```python
from build123d import *

# Parameters (mm, degrees)
F0_R     = 1.6
F0_R_2   = 1.7
F0_R_3   = 11.25
F1_DEPTH = 10
F2_R     = 2


# Not quite as in the source:
# - a feature of the source that left no trace in its solid (it failed there, or was rolled back) is left out


with BuildPart() as f1:
    # F0 (on Front) → F1 (new body)
    with BuildSketch(Plane.XZ):
        with BuildLine():
            Line((11.2397133785, 19.9999894063), (-11.2602985395, 19.9999894063))
            ThreePointArc((-11.2602985395, 19.9999894063), (-18.3350043941, 17.0674173026), (-21.2602932426, 9.9896968203))
            Line((-21.2602932426, 9.9896968203), (-21.229426084, -19.9999894063))
            Line((-21.229426084, -19.9999894063), (-43.3949531186, -19.9999894063))
            Line((-43.3949531186, -19.9999894063), (-43.3949531186, -29.9999894063))
            Line((-43.3949531186, -29.9999894063), (43.3949531186, -29.9999894063))
            Line((43.3949531186, -29.9999894063), (43.3949531186, -19.9999894063))
            Line((43.3949531186, -19.9999894063), (21.2705964277, -19.9999894063))
            Line((21.2705964277, -19.9999894063), (21.2397080816, 10.0102819922))
            ThreePointArc((21.2397080816, 10.0102819922), (18.3071412749, 17.0746952609), (11.2397133785, 19.9999894063))
        make_face()
        with Locations((-15.6323080096, -17.1999894063)):
            Circle(F0_R, mode=Mode.SUBTRACT)
        with Locations((15.6677115429, -17.1999961863)):
            Circle(F0_R, mode=Mode.SUBTRACT)
        with Locations((-15.6645237988, 14.0999894063)):
            Circle(F0_R_2, mode=Mode.SUBTRACT)
        Circle(F0_R_3, mode=Mode.SUBTRACT)
        with Locations((15.629426084, 14.0999894063)):
            Circle(F0_R, mode=Mode.SUBTRACT)
    extrude(amount=F1_DEPTH)

    # F2
    f2_edges = [f1.edges().sort_by_distance(p)[0] for p in [
        (21.270596, -5, -19.999989),
        (-21.229426, -5, -19.999989),
    ]]
    fillet(f2_edges, radius=F2_R)


solid = f1.part
```
For this review, take the finished solid that the model builds, in its own axes (mm). A direction names the side the tool comes from. Coordinates: 2 decimals unless noted, no trailing zeros. Order: outer loops, then holes, each group sorted by start corner. A loop starts at its lowest first (then second) coordinate and runs counter-clockwise, first axis right, second up. Notation, with made-up numbers: (82, 69) -> (128, 69) arc R20 cw to (128, 91) -> close; hole circle Ø3 at (7, -39.75). An arc over 180 degrees is marked (long way). Answer as CSV lines item,"result".
Q1. Wall thickness on line 1 along X through (y, z) = (-5.5, -0.5); line 2 along X through (y, z) = (-5.75, -18.5) (3 decimals); line 3 along Z through (x, y) = (-16, -0.5): over which ranges is each line inside the solid? List them lowest first. Write a range as [from, to].
Model answer:
line 1,"x = [-21.25, -11.24], [11.24, 21.25]"
line 2,"x = [-21.295, -16.565], [-14.7, 14.735], [16.6, 21.332]"
line 3,"z = [-30, -18.76], [-15.64, 12.43], [15.77, 18.81]"
Q2. Draft analysis for pull direction Z (two halves, no side actions). For faces 1 (the face through (-43.395, -5, -25)), 2 (the face through (0, -5, 20)), 3 (the face through (17.11, -4.93, 13.49)), 4 (the face through (-16.917, -4.93, 15.249)), state which applies: released by +Z, released by -Z, zero draft, split by the parting line, or undercut.
Model answer:
face 1,"zero draft"
face 2,"released by +Z"
face 3,"undercut"
face 4,"undercut"
Q3. For faces 5 (the face through (-1, -5, -30)), 6 (the face through (-33, -5, -20)), 7 (the face through (33, -5, -20)), list the 3-axis set-ups (+Z, -Z, +X, -X, +Y, -Y) from which the entire face can be reached by the end or side of a thin tool; tool diameter is ignored.
Model answer:
face 5,"-Z, +X, -X, +Y, -Y"
face 6,"+Z, -X, +Y, -Y"
face 7,"+Z, +X, +Y, -Y"
Q4. We need section D-D (x = -27.5). State the section outline as (y, z) points, plus the area to 3 significant figures.
Model answer:
outline,"(-10, -30) -> (0, -30) -> (0, -20) -> (-10, -20) -> close"
area,"100 mm2"
Q5. We need section C-C (y = -5.5). State the section outline as (x, z) points.
Model answer:
outline,"(-43.39, -30) -> (43.39, -30) -> (43.39, -20) -> (23.27, -20) arc R2 cw to (21.27, -18) -> (21.24, 10.01) arc R10 ccw to (11.24, 20) -> (-11.26, 20) arc R10 ccw to (-21.26, 9.99) -> (-21.23, -18) arc R2 cw to (-23.23, -20) -> (-43.39, -20) -> close; hole circle Ø3.4 at (-15.66, 14.1); hole circle Ø3.2 at (-15.63, -17.2); hole circle Ø22.5 at (0, 0); hole circle Ø3.2 at (15.63, 14.1); hole circle Ø3.2 at (15.67, -17.2)"
Q6. Clearance check with flat-ended pins moving along their axes: pin 1 Ø6 at (x, y) = (22, -3) entering from +Z; pin 2 Ø20 at (x, z) = (0, 0) entering from +Y; pin 3 Ø1.5 at (y, z) = (-9, 5) entering from +X. State where each tip first meets the part, or that it passes through.
Model answer:
pin 1,"stops at z = 16.31"
pin 2,"passes through"
pin 3,"stops at x = 21.25"
Q7. We need section B-B (z = 0). State the section outline as (x, y) points.
Model answer:
outline,"(-21.25, -10) -> (-11.25, -10) -> (-11.25, 0) -> (-21.25, 0) -> close; (11.25, -10) -> (21.25, -10) -> (21.25, 0) -> (11.25, 0) -> close"
Q8. We need section A-A (x = 0). State the section outline as (y, z) points.
Model answer:
outline,"(-10, -30) -> (0, -30) -> (0, -11.25) -> (-10, -11.25) -> close; (-10, 11.25) -> (0, 11.25) -> (0, 20) -> (-10, 20) -> close"
